from build123d import *

# Parameters (mm, degrees)
SKETCH_1_R          = 2
EXTRUDE_1_DEPTH     = 160
SKETCH_3_R          = 20
EXTRUDE_2_DEPTH     = 2
SKETCH_4_R          = 2
CUT_EXTRUDE_1_DEPTH = 2
EXTRUDE_3_DEPTH     = 100


with BuildPart() as part:
    # 草图1 → 凸台-拉伸1 (new body)
    with BuildSketch(Plane.XY):
        Circle(SKETCH_1_R)
    extrude(amount=EXTRUDE_1_DEPTH)

    # 草图3 → 凸台-拉伸2 (add)
    with BuildSketch(Plane(origin=(0, 0, 0), x_dir=(-1, 0, 0), z_dir=(0, 0, -1))):
        Circle(SKETCH_3_R)
    extrude(amount=-EXTRUDE_2_DEPTH)

    # 草图4 → 切除-拉伸1 (cut)
    with BuildSketch(Plane(origin=(0, 0, 0), x_dir=(-1, 0, 0), z_dir=(0, 0, -1))):
        with Locations((0, 17.25)):
            Circle(SKETCH_4_R)
        with Locations((14.938938215, 8.625)):
            Circle(SKETCH_4_R)
        with Locations((14.938938215, -8.625)):
            Circle(SKETCH_4_R)
        with Locations((0, -17.25)):
            Circle(SKETCH_4_R)
        with Locations((-14.938938215, -8.625)):
            Circle(SKETCH_4_R)
        with Locations((-14.938938215, 8.625)):
            Circle(SKETCH_4_R)
    extrude(amount=-CUT_EXTRUDE_1_DEPTH, mode=Mode.SUBTRACT)

    # 草图5 → 凸台-拉伸3 (add)
    with BuildSketch(Plane.XY.offset(160)):
        Polygon((-2.419835519, 0), (-2.419835519, 0.625), (-1.899835519, 0.625), (-1.899835519, -0.625), (-2.419835519, -0.625), align=None)
    extrude(amount=-EXTRUDE_3_DEPTH)


solid = part.part
The listing builds one solid part. Answer for the finished solid, in the listing's coordinates (mm). Round coordinates to 2 decimals unless told otherwise and drop trailing zeros. Loops run counter-clockwise (first coordinate to the right, second up) from the corner with the lowest first, then second, coordinate; pieces in that order, holes last. Notation, with made-up numbers: M 39,83 L 58,83 A22 ccw 58,113 Z; hole C 39.25,33.25 d7. An arc over 180 degrees is marked long. Write each question's results on one line, items separated by ' | '. Start each with the question number.
1) Find section C-C on z = 22.5. Write down the section's boundary in (x, y).
2) Find section B-B on y = -17.25. Write down the section's boundary in (x, z).
3) Straight lines are drawn through the part: probe 1 along Z at (x, y) = (13, 2.5); probe 2 along Y at (x, z) = (-2, 75.5) (3 decimals); probe 3 along Y at (x, z) = (1, 47.5). For each, find the intervals that lie inside material, in ascending order.
4) Find section A-A on x = 0. Write down the section's boundary in (y, z).
5) Determine the mould class of faces 1 (the cylindrical face through (0.26, 19.233, 0.986)), 2 (the cylindrical face through (1.908, 0.601, 79.894)), 3 (the flat face through (0, -4, 2)) for opening direction X: pulls with the +X half, pulls with the -X half, needs draft (parallel to the pull), parting line crosses it, or undercut.
6) Each of these flat-tipped pins is pushed along its axis until it touches: pin 1 (2.5 mm diameter, centred on x = 0, y = 17.25, fed in from +Z); pin 2 (12 mm diameter, centred on x = 5, y = 9.5, fed in from +Z). Where does it stop, or does it pass through?
7) Find section D-D on x = 7. Write down the section's boundary in (y, z) (3 decimals).
Final values:
1) outline: C 0,0 d4
2) outline: M -10.12,0 L -2,0 L -2,2 L -10.12,2 Z; M 2,0 L 10.12,0 L 10.12,2 L 2,2 Z
3) probe 1: 0 to 2 | probe 2: -0.625 to 0.625 | probe 3: -1.73 to 1.73
4) outline: M -20,0 L -19.25,0 L -19.25,2 L -20,2 Z; M -15.25,0 L 15.25,0 L 15.25,2 L 2,2 L 2,160 L -2,160 L -2,2 L -15.25,2 Z; M 19.25,0 L 20,0 L 20,2 L 19.25,2 Z
5) face 1: undercut | face 2: parting line crosses it | face 3: needs draft
6) pin 1: through | pin 2: z = 2
7) outline: M -18.735,0 L 18.735,0 L 18.735,2 L -18.735,2 Z
